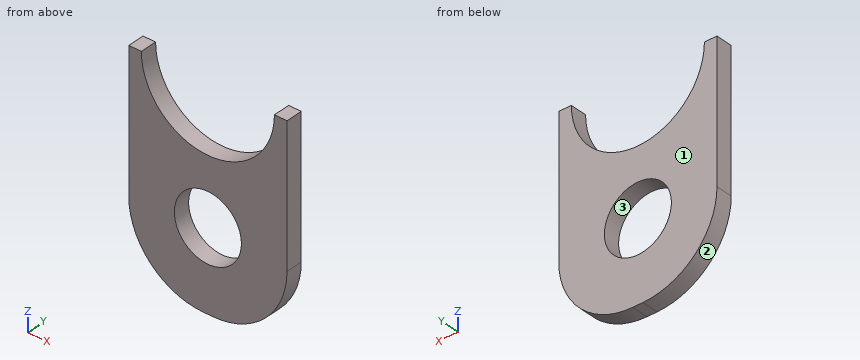
```python
from build123d import *

# Parameters (mm, degrees)
SKETCH1_R           = 8
BOSS_EXTRUDE1_DEPTH = 4


with BuildPart() as part:
    # Sketch1 → Boss-Extrude1 (new body)
    with BuildSketch(Plane(origin=(0, 0, 0), x_dir=(1, 0, 0), z_dir=(0, 1, 0))):
        with BuildLine():
            Line((0, 0), (-3, 0))
            ThreePointArc((-3, 0), (-18.88, 15.88), (-34.76, 0))
            Line((-34.76, 0), (-37.76, 0))
            Line((-37.76, 0), (-37.76, 33.101))
            ThreePointArc((-37.76, 33.101), (-32.57608292, 45.61608292), (-20.061, 50.8))
            Line((-20.061, 50.8), (-17.699, 50.8))
            ThreePointArc((-17.699, 50.8), (-5.18391708, 45.61608292), (0, 33.101))
            Line((0, 33.101), (0, 0))
        make_face()
        with Locations(Location((-18.88, 31.8, 0), (0, 0, 270))):
            Circle(SKETCH1_R, mode=Mode.SUBTRACT)
    extrude(amount=BOSS_EXTRUDE1_DEPTH)


solid = part.part
```
Design review of the part built by this model. Coordinates are the model's own, in mm. Face numbers are marked on the shaded views. Give positions to 0.01 mm unless a question says otherwise; leave off trailing zeros. Write each loop counter-clockwise with the first axis right and the second up, starting at its lowest first coordinate (ties: lowest second). Pieces come first, ordered by that corner, then holes. Notation, with made-up numbers: (41, 11.25) - (71, 11.25) arc R12 ccw to (71, 26.25) - close; hole circle Ø8 at (31, 76.5). An arc over 180 degrees is marked (long way). Return JSON: item names as keys, results as strings. Group by question number.
(1) We need section B-B, the plane x = -18.88. Give the boundary of the cut face in (y, z), then the cut area to 3 significant figures.
(2) To check wall thickness, follow probe 1 along X at (y, z) = (2.4, -31.8); probe 2 along X at (y, z) = (2.75, -31); probe 3 along Z at (x, y) = (-15, 3.85). State the ranges of each line that lie inside material, in increasing order.
(3) We need section A-A, the plane z = -31.8. Give the boundary of the cut face in (x, y), then the cut area to 3 significant figures.
(4) We need section D-D, the plane x = -5. Give the boundary of the cut face in (y, z).
(5) We need section C-C, the plane y = 2.75. Give the boundary of the cut face in (x, z).
(6) Insertion check: pin 1 (13 mm diameter, centred on x = -18.88, z = -31.8, fed in from +Y). The pin has a flat end and moves straight along its axis. Give the tip position at first contact, or say it passes through.
(7) Mouldability with a two-part tool opening along X and no side actions: class the marked faces 1, 2 and 3 as +X half, -X half, draft (parallel to the pull), parting line (faces both ways), or undercut.
Reported:
{
 "1": {"outline": "(0, -50.8) - (4, -50.8) - (4, -39.8) - (0, -39.8) - close; (0, -23.8) - (4, -23.8) - (4, -15.88) - (0, -15.88) - close", "area": "75.7 mm2"},
 "2": {"probe 1": "x = -37.76 to -26.88, -10.88 to 0", "probe 2": "x = -37.76 to -26.84, -10.92 to 0", "probe 3": "z = -50.59 to -38.8, -24.8 to -15.4"},
 "3": {"outline": "(-37.76, 0) - (-26.88, 0) - (-26.88, 4) - (-37.76, 4) - close; (-10.88, 0) - (0, 0) - (0, 4) - (-10.88, 4) - close", "area": "87.0 mm2"},
 "4": {"outline": "(0, -45.43) - (4, -45.43) - (4, -7.71) - (0, -7.71) - close"},
 "5": {"outline": "(-37.76, -33.1) arc R17.7 ccw to (-20.06, -50.8) - (-17.7, -50.8) arc R17.7 ccw to (0, -33.1) - (0, 0) - (-3, 0) arc R15.88 cw to (-34.76, 0) - (-37.76, 0) - close; hole circle Ø16 at (-18.88, -31.8)"},
 "6": {"pin 1": "passes through"},
 "7": {"face 1": "draft", "face 2": "-X half", "face 3": "undercut"}
}
